from build123d import *

# Parameters (mm, degrees)
EXTRUDE_1_DEPTH     = 3
SKETCH_2_R          = 1.15
CUT_EXTRUDE_1_DEPTH = 326.052303484


with BuildPart() as part:
    # 草图1 → 凸台-拉伸1 (new body)
    with BuildSketch(Plane.XY):
        Polygon((0, 0), (10, 5), (315, 5), (325, 0), (315, 0), (315, -3), (290, -3), (290, 0), (280, 0), (280, -3), (255, -3), (255, 0), (245, 0), (245, -3), (220, -3), (220, 0), (210, 0), (210, -3), (185, -3), (185, 0), (175, 0), (175, -3), (150, -3), (150, 0), (140, 0), (140, -3), (115, -3), (115, 0), (105, 0), (105, -3), (80, -3), (80, 0), (70, 0), (70, -3), (45, -3), (45, 0), (35, 0), (35, -3), (10, -3), (10, 0), align=None)
    extrude(amount=EXTRUDE_1_DEPTH)

    # 草图2 → 切除-拉伸1 (cut, through all)
    with BuildSketch(Plane.XY.offset(3)):
        with Locations((22.5, 2.85)):
            Circle(SKETCH_2_R)
        with Locations((57.5, 2.85)):
            Circle(SKETCH_2_R)
        with Locations((92.5, 2.85)):
            Circle(SKETCH_2_R)
        with Locations((127.5, 2.85)):
            Circle(SKETCH_2_R)
        with Locations((162.5, 2.85)):
            Circle(SKETCH_2_R)
        with Locations((197.5, 2.85)):
            Circle(SKETCH_2_R)
        with Locations((232.5, 2.85)):
            Circle(SKETCH_2_R)
        with Locations((267.5, 2.85)):
            Circle(SKETCH_2_R)
        with Locations((302.5, 2.85)):
            Circle(SKETCH_2_R)
    extrude(amount=-CUT_EXTRUDE_1_DEPTH, mode=Mode.SUBTRACT)


solid = part.part
Can you work these out from the model? Positions are in its coordinate system, mm. Give positions to 0.01 mm unless a question says otherwise; leave off trailing zeros. Return JSON: item names as keys, results as strings.
1. I'm going to push flat-ended pins straight in: pin 1 Ø0.9 at (y, z) = (-1.5, 1.5) entering from +X; pin 2 Ø1.5 at (y, z) = (-2, 1.5) entering from -X; pin 3 Ø1.5 at (x, z) = (73, 2) entering from -Y. Where does each tip first touch, or does it pass through?
Output values:
{"pin 1": "stops at x = 315", "pin 2": "stops at x = 10", "pin 3": "stops at y = 0"}
2. If I drill on line 1 (Y direction, x = 162.5, z = 2.2); line 2 (Y direction, x = 127, z = 1); line 3 (Y direction, x = 37.5, z = 1.05), over which ranges is the centre line in solid material (lowest first)?
Output values:
{"line 1": "y = -3 to 1.7, 4 to 5", "line 2": "y = -3 to 1.81, 3.89 to 5", "line 3": "y = 0 to 5"}
3. I want a section at A-A on y = -1.25. Give the number of separate pieces and of enclosed holes in the cut face, and give its area (3 significant figures).
Output values:
{"separate pieces": "9", "enclosed holes": "0", "area": "675 mm²"}
